```python
from build123d import *

# Parameters (mm, degrees)
F1_ANGLE  = 90
F3_COUNT  = 4
F3_ANGLE  = 270
F9_ANGLE  = 90
F10_COUNT = 4
F10_ANGLE = 270
F13_COUNT = 2
F13_ANGLE = 90


with BuildPart() as f1:
    # F0 (on Top) → F1 (revolve)
    with BuildSketch(Plane.XY):
        with BuildLine():
            Line((-36.83, 36.83), (-36.83, 4.445))
            ThreePointArc((-36.83, 4.445), (-13.9303468913, 13.9303468913), (-4.445, 36.83))
            Line((-4.445, 36.83), (-36.83, 36.83))
        make_face()
    revolve(axis=Axis((-36.83, 20.6375, 0), (0, -1, 0)), revolution_arc=F1_ANGLE)


with BuildPart() as f3_1:
    # F3: instance of F1
    add(f1.part.rotate(Axis((0, 0, 12.7), (0, 0, 1)), 1 * F3_ANGLE / (F3_COUNT - 1)))


with BuildPart() as f3_2:
    # F3: instance of F1
    add(f1.part.rotate(Axis((0, 0, 12.7), (0, 0, 1)), 2 * F3_ANGLE / (F3_COUNT - 1)))


with BuildPart() as f3_3:
    # F3: instance of F1
    add(f1.part.rotate(Axis((0, 0, 12.7), (0, 0, 1)), 3 * F3_ANGLE / (F3_COUNT - 1)))


with BuildPart() as f5_1:
    # F5: instance of F1
    add(f1.part.mirror(Plane.XY.offset(36.83)))


with BuildPart() as f5_2:
    # F5: instance of F3_1
    add(f3_1.part.mirror(Plane.XY.offset(36.83)))


with BuildPart() as f5_3:
    # F5: instance of F3_2
    add(f3_2.part.mirror(Plane.XY.offset(36.83)))


with BuildPart() as f5_4:
    # F5: instance of F3_3
    add(f3_3.part.mirror(Plane.XY.offset(36.83)))


with BuildPart() as f7:
    # F6 (on offset) → F7 (revolve)
    with BuildSketch(Plane.XY.offset(36.83)):
        with BuildLine():
            Line((32.639, 0), (-32.639, 0))
            ThreePointArc((-32.639, 0), (0, -32.639), (32.639, 0))
        make_face()
    revolve(axis=Axis((0, 0, 36.83), (1, 0, 0)))


with BuildPart() as f9:
    # F8 (on Top) → F9 (revolve)
    with BuildSketch(Plane.XY):
        with BuildLine():
            Line((4.6355, 36.83), (-4.6355, 36.83))
            ThreePointArc((-4.6355, 36.83), (0, 32.1945), (4.6355, 36.83))
        make_face()
    revolve(axis=Axis((0, 36.83, 0), (-1, 0, 0)), revolution_arc=F9_ANGLE)


with BuildPart() as f10_1:
    # F10: instance of F9
    add(f9.part.rotate(Axis((0, 0, 12.7), (0, 0, 1)), 1 * F10_ANGLE / (F10_COUNT - 1)))


with BuildPart() as f10_2:
    # F10: instance of F9
    add(f9.part.rotate(Axis((0, 0, 12.7), (0, 0, 1)), 2 * F10_ANGLE / (F10_COUNT - 1)))


with BuildPart() as f10_3:
    # F10: instance of F9
    add(f9.part.rotate(Axis((0, 0, 12.7), (0, 0, 1)), 3 * F10_ANGLE / (F10_COUNT - 1)))


with BuildPart() as f11_1:
    # F11: instance of F9
    add(f9.part.mirror(Plane.XY.offset(36.83)))


with BuildPart() as f11_2:
    # F11: instance of F10_3
    add(f10_3.part.mirror(Plane.XY.offset(36.83)))


with BuildPart() as f11_3:
    # F11: instance of F10_2
    add(f10_2.part.mirror(Plane.XY.offset(36.83)))


with BuildPart() as f11_4:
    # F11: instance of F10_1
    add(f10_1.part.mirror(Plane.XY.offset(36.83)))


with BuildPart() as f13_1:
    # F13: instance of F9
    add(f9.part.rotate(Axis((0, 12.7, 36.83), (0, 1, 0)), 1 * F13_ANGLE / (F13_COUNT - 1)))


with BuildPart() as f13_2:
    # F13: instance of F10_2
    add(f10_2.part.rotate(Axis((0, 12.7, 36.83), (0, 1, 0)), 1 * F13_ANGLE / (F13_COUNT - 1)))


with BuildPart() as f1_1:
    add(f1.part)

    add(f3_1.part)  # F14 merges F3_1

    add(f3_2.part)  # F14 merges F3_2

    add(f3_3.part)  # F14 merges F3_3

    add(f5_1.part)  # F14 merges F5_1

    add(f5_2.part)  # F14 merges F5_2

    add(f5_3.part)  # F14 merges F5_3

    add(f5_4.part)  # F14 merges F5_4

    add(f7.part)  # F14 merges F7

    add(f9.part)  # F14 merges F9

    add(f10_1.part)  # F14 merges F10_1

    add(f10_2.part)  # F14 merges F10_2

    add(f10_3.part)  # F14 merges F10_3

    add(f11_1.part)  # F14 merges F11_1

    add(f11_2.part)  # F14 merges F11_2

    add(f11_3.part)  # F14 merges F11_3

    add(f11_4.part)  # F14 merges F11_4

    add(f13_1.part)  # F14 merges F13_1

    add(f13_2.part)  # F14 merges F13_2
    # F14: F13_1, F13_2 across plane
    add(f13_1.part.mirror(Plane.YZ))
    add(f13_2.part.mirror(Plane.YZ))


solid = f1_1.part
```
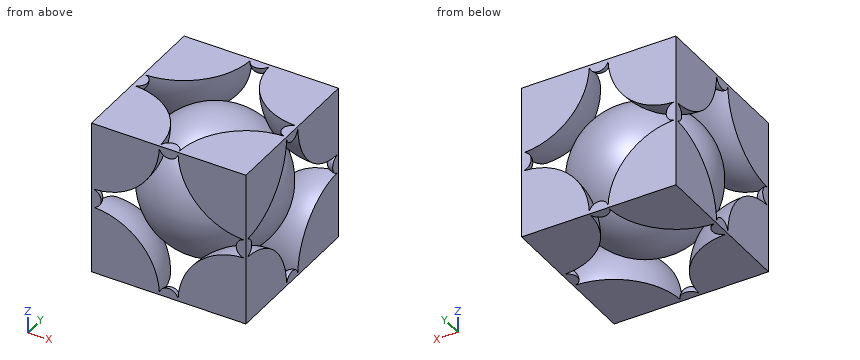
Design review of the part built by this model. Coordinates are the model's own, in mm. Round coordinates to 2 decimals unless told otherwise and drop trailing zeros. Order: outer loops, then holes, each group sorted by start corner. A loop starts at its lowest first (then second) coordinate and runs counter-clockwise, first axis right, second up. Notation, with made-up numbers: M 83.25,54 L 104.25,54 A9 cw 104.25,68 Z; hole C 35,55 d11. An arc over 180 degrees is marked long. Put each result on its own line as item: value.
Q1. Consider section B-B (y = 7). State the section outline as (x, z) points.
Reported:
outline: M -36.83,0 L -24.22,0 A12.61 ccw -36.83,12.61 Z; M -36.83,61.05 A12.61 ccw -24.22,73.66 L -36.83,73.66 Z; C 0,36.83 d63.76; M 24.22,0 L 36.83,0 L 36.83,12.61 A12.61 ccw Z; M 24.22,73.66 A12.61 ccw 36.83,61.05 L 36.83,73.66 Z
Q2. To check wall thickness, follow line 1 (Y direction, x = -23, z = 5.5); line 2 (Y direction, x = -18, z = 61); line 3 (X direction, y = 19.5, z = 60). State the ranges of each line that lie inside material, in increasing order.
Reported:
line 1: -36.83 to -8.07, 8.07 to 36.83
line 2: -36.83 to -13.72, -12.53 to 12.53, 13.72 to 36.83
line 3: -36.83 to -13.13, -12.17 to 12.17, 13.13 to 36.83
Q3. Consider section A-A (x = -11.5). State the section outline as (y, z) points.
Reported:
outline: M -36.83,0 L -16.65,0 A20.18 ccw -36.83,20.18 Z; M -36.83,53.48 A20.18 ccw -16.65,73.66 L -36.83,73.66 Z; C 0,36.83 d61.09; M 16.65,0 L 36.83,0 L 36.83,20.18 A20.18 ccw Z; M 16.65,73.66 A20.18 ccw 36.83,53.48 L 36.83,73.66 Z
Q4. Consider section C-C (z = 14). State the section outline as (x, y) points, and give its area (3 significant figures).
Reported:
outline: M -36.83,-36.83 L -7.63,-36.83 A29.2 ccw -13.93,-18.71 A23.33 ccw 13.93,-18.71 A29.2 ccw 7.63,-36.83 L 36.83,-36.83 L 36.83,-7.63 A29.2 ccw 18.71,-13.93 A23.33 ccw 18.71,13.93 A29.2 ccw 36.83,7.63 L 36.83,36.83 L 7.63,36.83 A29.2 ccw 13.93,18.71 A23.33 ccw -13.93,18.71 A29.2 ccw -7.63,36.83 L -36.83,36.83 L -36.83,7.63 A29.2 ccw -18.71,13.93 A23.33 ccw -18.71,-13.93 A29.2 ccw -36.83,-7.63 Z
area: 4,380 mm²
Q5. Insertion check: pin 1 Ø8 at (y, z) = (-12, 47) entering from -X; pin 2 Ø2 at (x, y) = (-4, 8.5) entering from -Z; pin 3 Ø1 at (x, y) = (-22, -5) entering from -Z. Each pin has a flat end and moves straight along its axis. Give the tip position at first contact, or say it passes through.
Reported:
pin 1: x = -30.46
pin 2: z = 5.29
pin 3: z = 12.78
Q6. Consider section D-D (y = 19). State the section outline as (x, z) points, and give its area (3 significant figures).
Reported:
outline: M -36.83,0 L -9.8,0 A27.03 ccw -13.8,14.16 A26.54 ccw 13.8,14.16 A27.03 ccw 9.8,0 L 36.83,0 L 36.83,27.03 A27.03 ccw 22.67,23.03 A26.54 ccw 22.67,50.63 A27.03 ccw 36.83,46.63 L 36.83,73.66 L 9.8,73.66 A27.03 ccw 13.8,59.5 A26.54 ccw -13.8,59.5 A27.03 ccw -9.8,73.66 L -36.83,73.66 L -36.83,46.63 A27.03 ccw -22.67,50.63 A26.54 ccw -22.67,23.03 A27.03 ccw -36.83,27.03 Z
area: 4,460 mm²
